```python
from build123d import *

# Parameters (mm, degrees)
SKETCH1_W           = 10
SKETCH1_H           = 3
BOSS_EXTRUDE1_DEPTH = 3
SKETCH2_W           = 3
SKETCH2_H           = 5
CUT_EXTRUDE1_DEPTH  = 3


with BuildPart() as part:
    # Sketch1 → Boss-Extrude1 (new body)
    with BuildSketch(Plane.XY):
        Polygon((-3.827421787, 35.839698152), (-13.827421787, 35.839698152), (-16.25, 35.839698152), (-19.25, 35.839698152), (-19.25, 25.839698152), (-13.827421787, 25.839698152), (-3.827421787, 25.839698152), (3.672578213, 25.839698152), (13.672578213, 25.839698152), (19.25, 25.839698152), (19.25, 35.839698152), (16.25, 35.839698152), (13.672578213, 35.839698152), (3.672578213, 35.839698152), align=None)
        with Locations((-8.827421787, 37.339698152)):
            Rectangle(SKETCH1_W, SKETCH1_H)
        with Locations((8.672578213, 37.339698152)):
            Rectangle(SKETCH1_W, SKETCH1_H)
        with Locations((-8.827421787, 24.339698152)):
            Rectangle(SKETCH1_W, SKETCH1_H)
        with Locations((8.672578213, 24.339698152)):
            Rectangle(SKETCH1_W, SKETCH1_H)
    extrude(amount=BOSS_EXTRUDE1_DEPTH)

    # Sketch2 → Cut-Extrude1 (cut)
    with BuildSketch(Plane.XY.offset(3)):
        with Locations((-17.75, 30.839698152)):
            Rectangle(SKETCH2_W, SKETCH2_H)
        with Locations((17.75, 30.839698152)):
            Rectangle(SKETCH2_W, SKETCH2_H)
    extrude(amount=-CUT_EXTRUDE1_DEPTH, mode=Mode.SUBTRACT)


solid = part.part
```
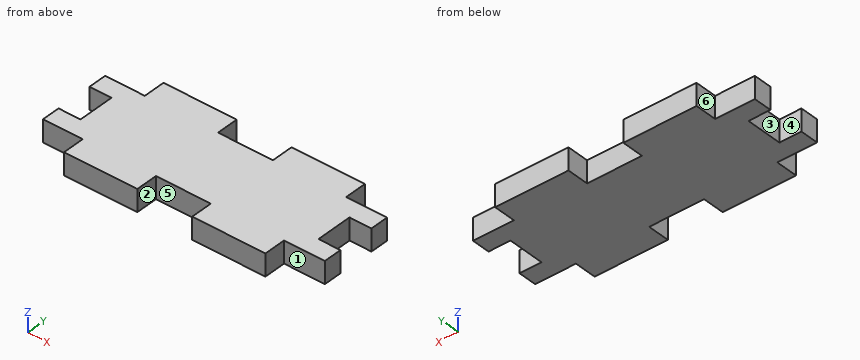
Could you check a few things on this model? Use its own coordinates, in mm. Face numbers are marked on the shaded views. A direction names the side the tool comes from. Coordinates: 2 decimals unless noted, no trailing zeros. Write each loop counter-clockwise with the first axis right and the second up, starting at its lowest first coordinate (ties: lowest second). Pieces come first, ordered by that corner, then holes. Notation, with made-up numbers: (-2.5, -36) -> (7.5, -36) arc R15 ccw to (7.5, -21) -> close; hole circle Ø8 at (51, -4). An arc over 180 degrees is marked (long way). One line per question, with ' | ' between items. Start each with the question number.
1. If we section it at A-A (y = 37): Please give me the cut outline in (x, z), and give its area (3 significant figures).
2. If we section it at B-B (z = 0.8): Please give me the cut outline in (x, y), and give its area (3 significant figures).
3. If we section it at C-C (x = -0.5): Please give me the cut outline in (y, z), and give its area (3 significant figures).
4. Will these pins go through, and if not, where does the flat tip stop? P1, Ø1, axis at y = 36, z = 1.5, coming from the +X side; P2, Ø0.9, axis at y = 38, z = 1.5, coming from the +X side; P3, Ø0.9, axis at y = 25, z = 1, coming from the -X side; P4, Ø1.5, axis at x = -17, z = 1, coming from the -Y side.
5. Please list where these lines run through material, in increasing order: line 1 along Y through (x, z) = (18.5, 2.2); line 2 along X through (y, z) = (24.25, 2.7); line 3 along Y through (x, z) = (2, 2).
6. Thinking about a two-plate mould opening in X: for the marked faces 1, 2 and 3, which applies, pulls with the +X half, pulls with the -X half, needs draft (parallel to the pull), parting line crosses it, or undercut?
7. If we section it at D-D (y = 31): Please give me the cut outline in (x, z).
8. For the marked faces 4, 5 and 6, which set-ups out of +Z, -Z, +X, -X, +Y, -Y let a thin tool reach every point of the face, with its end or its side?
Return value:
1) outline: (-13.83, 0) -> (-3.83, 0) -> (-3.83, 3) -> (-13.83, 3) -> close; (3.67, 0) -> (13.67, 0) -> (13.67, 3) -> (3.67, 3) -> close | area: 60.0 mm²
2) outline: (-19.25, 25.84) -> (-13.83, 25.84) -> (-13.83, 22.84) -> (-3.83, 22.84) -> (-3.83, 25.84) -> (3.67, 25.84) -> (3.67, 22.84) -> (13.67, 22.84) -> (13.67, 25.84) -> (19.25, 25.84) -> (19.25, 28.34) -> (16.25, 28.34) -> (16.25, 33.34) -> (19.25, 33.34) -> (19.25, 35.84) -> (13.67, 35.84) -> (13.67, 38.84) -> (3.67, 38.84) -> (3.67, 35.84) -> (-3.83, 35.84) -> (-3.83, 38.84) -> (-13.83, 38.84) -> (-13.83, 35.84) -> (-19.25, 35.84) -> (-19.25, 33.34) -> (-16.25, 33.34) -> (-16.25, 28.34) -> (-19.25, 28.34) -> close | area: 475 mm²
3) outline: (25.84, 0) -> (35.84, 0) -> (35.84, 3) -> (25.84, 3) -> close | area: 30.0 mm²
4) P1: stops at x = 19.25 | P2: stops at x = 13.67 | P3: stops at x = -13.83 | P4: stops at y = 25.84
5) line 1: y = 25.84 to 28.34, 33.34 to 35.84 | line 2: x = -13.83 to -3.83, 3.67 to 13.67 | line 3: y = 25.84 to 35.84
6) face 1: needs draft | face 2: undercut | face 3: pulls with the -X half
7) outline: (-16.25, 0) -> (16.25, 0) -> (16.25, 3) -> (-16.25, 3) -> close
8) face 4: +Z, -Z, -X | face 5: +Z, -Z, -Y | face 6: +Z, -Z, -X, +Y
